Work out the finished part from the listing and answer in its coordinate system (mm). Round coordinates to 2 decimals unless told otherwise and drop trailing zeros. Write each loop counter-clockwise with the first axis right and the second up, starting at its lowest first coordinate (ties: lowest second). Pieces come first, ordered by that corner, then holes. Notation, with made-up numbers: M 20,-0.5 L 54,-0.5 A28 ccw 54,24.5 Z; hole C 36.25,-19 d2. An arc over 180 degrees is marked long. Answer in a Markdown table with one row per item.
```python
from build123d import *

# Parameters (mm, degrees)
BOSS_EXTRUDE2_DEPTH = 3
SKETCH4_R           = 2
CUT_EXTRUDE2_DEPTH  = 3


with BuildPart() as part:
    # Sketch3 → Boss-Extrude2 (new body)
    with BuildSketch(Plane(origin=(0, 0, 0), x_dir=(1, 0, 0), z_dir=(0, 1, 0))):
        with BuildLine():
            ThreePointArc((0, 20.000004284), (-15.361487959, -4.421029535), (10.567709202, 8.229620236))
            add(Edge.make_bspline(
                [(10.567709202, 8.229620236), (43.206989346, 32.255448903), (82.778918939, 49.08436074), (129.283499892, 58.71635639)],
                knots=[0.095561107, 0.095561107, 0.095561107, 0.095561107, 0.960221945, 0.960221945, 0.960221945, 0.960221945], degree=3))
            add(Edge.make_bspline(
                [(135.745739898, 54), (134.188411223, 58.347154687), (129.283499892, 58.71635639)],
                knots=[0, 0, 0, 1, 1, 1], degree=2))
            Line((135.745739898, 54), (135.745739898, 65))
            Line((135.745739898, 65), (132.745739898, 65))
            Line((132.745739898, 65), (132.745739898, 75))
            Line((132.745739898, 75), (135.745739898, 75))
            Line((135.745739898, 75), (135.745739898, 85))
            add(Edge.make_bspline(
                [(135.745739898, 85), (134.392955154, 81.542928592), (129.283499131, 78.716356348)],
                knots=[0, 0, 0, 1, 1, 1], degree=2))
            add(Edge.make_bspline(
                [(0, 20.000004284), (34.544798533, 48.4477318), (77.639296954, 68.019848628), (129.283499131, 78.716356348)],
                knots=[0, 0, 0, 0, 0.960221944, 0.960221944, 0.960221944, 0.960221944], degree=3))
        make_face()
    extrude(amount=BOSS_EXTRUDE2_DEPTH)

    # Sketch4 → Cut-Extrude2 (cut)
    with BuildSketch(Plane(origin=(0, 3, 0), x_dir=(1, 0, 0), z_dir=(0, 1, 0))):
        with Locations(Location((-4.199995888, 5.600003084, 0), (0, 0, 270))):
            Circle(SKETCH4_R)
    extrude(amount=-CUT_EXTRUDE2_DEPTH, mode=Mode.SUBTRACT)


solid = part.part
```
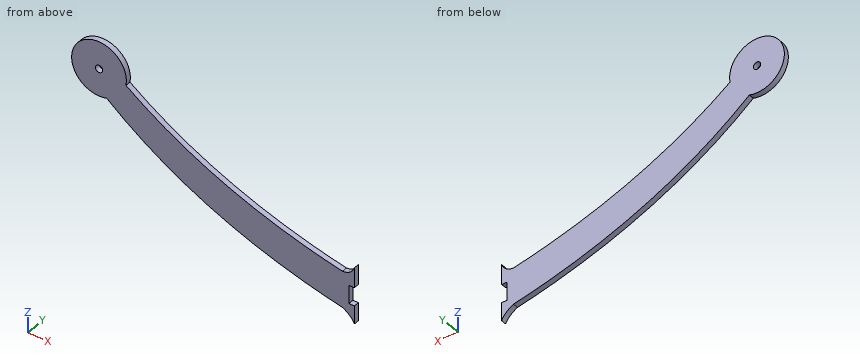
1. Consider line 1 along X through (y, z) = (0.2, 3); line 2 along Z through (x, y) = (81, 1.5); line 3 along X through (y, z) = (1.9, -30). Determine where each line is inside the solid, lowest interval first. Write a range as from..to.
Calculated:
| item | result |
|---|---|
| line 1 | x = -16.49..8.09 |
| line 2 | z = -65.25..-45.25 |
| line 3 | x = 13..45.8 |
2. The part is cut by section A-A (z = 3). Determine the outline of the cut face in (x, y).
Calculated:
| item | result |
|---|---|
| outline | M -16.49,0 L 8.09,0 L 8.09,3 L -16.49,3 Z |
3. Given pin 1 (6.5 mm diameter, centred on x = -4.2, z = -5.6, fed in from -Y); pin 2 (1.5 mm diameter, centred on y = 2, z = -12, fed in from +X), each flat-ended and moving along its own axis, determine where each tip first touches the part or whether it passes through.
Calculated:
| item | result |
|---|---|
| pin 1 | stops at y = 0 |
| pin 2 | stops at x = 16.91 |
